from build123d import *

# Parameters (mm, degrees)
SKETCH_1_R          = 22.5
EXTRUDE_1_DEPTH     = 3
SKETCH_2_R          = 22.5
SKETCH_2_R_2        = 21
EXTRUDE_2_DEPTH     = 9
SKETCH_4_R          = 4.1
SKETCH_4_R_2        = 1.5
CUT_EXTRUDE_1_DEPTH = 35.007352146


with BuildPart() as part:
    # 草图1 → 凸台-拉伸1 (new body)
    with BuildSketch(Plane.XY):
        Circle(SKETCH_1_R)
    extrude(amount=EXTRUDE_1_DEPTH)

    # 草图2 → 凸台-拉伸2 (add)
    with BuildSketch(Plane.XY.offset(3)):
        Circle(SKETCH_2_R)
        Circle(SKETCH_2_R_2, mode=Mode.SUBTRACT)
    extrude(amount=EXTRUDE_2_DEPTH)

    # 草图4 → 切除-拉伸1 (cut, through all)
    with BuildSketch(Plane(origin=(0, 0, 0), x_dir=(-1, 0, 0), z_dir=(0, 0, -1))):
        Circle(SKETCH_4_R)
        with Locations((0, 6.5)):
            Circle(SKETCH_4_R_2)
        with Locations((0, -6.5)):
            Circle(SKETCH_4_R_2)
    extrude(amount=-CUT_EXTRUDE_1_DEPTH, mode=Mode.SUBTRACT)


solid = part.part
For this review, take the finished solid that the model builds, in its own axes (mm). A direction names the side the tool comes from. Round coordinates to 2 decimals unless told otherwise and drop trailing zeros. Loops run counter-clockwise (first coordinate to the right, second up) from the corner with the lowest first, then second, coordinate; pieces in that order, holes last. Notation, with made-up numbers: (5, -35) - (20, -35) arc R22 ccw to (20, -8) - close; hole circle Ø7 at (-1.75, 69.25). An arc over 180 degrees is marked (long way). Answer as CSV lines item,"result".
(1) Wall thickness on line 1 (Y direction, x = 0, z = 0.7); line 2 (Z direction, x = 0, y = -12); line 3 (Y direction, x = 0, z = 7.75): over which ranges is each line inside the solid? List them lowest first.
Checked values:
line 1,"y = -22.5 to -8, -5 to -4.1, 4.1 to 5, 8 to 22.5"
line 2,"z = 0 to 3"
line 3,"y = -22.5 to -21, 21 to 22.5"
(2) Consider section A-A on y = 0. Give the boundary of the cut face in (x, z).
Checked values:
outline,"(-22.5, 0) - (-4.1, 0) - (-4.1, 3) - (-21, 3) - (-21, 12) - (-22.5, 12) - close; (4.1, 0) - (22.5, 0) - (22.5, 12) - (21, 12) - (21, 3) - (4.1, 3) - close"
(3) Insertion check: P1, Ø6, axis at x = -3.5, z = 8, coming from the -Y side; P2, Ø6, axis at y = 7.5, z = 6.5, coming from the -X side; P3, Ø1, axis at x = 3, z = 8, coming from the -Y side. Each pin has a flat end and moves straight along its axis. Give the tip position at first contact, or say it passes through.
Checked values:
P1,"stops at y = -22.49"
P2,"stops at x = -22.05"
P3,"stops at y = -22.36"
(4) Tool access review of faces 4 (the face through (4.4, 0.3, 3)), 5 (the face through (0, 5, 1)): name each direction out of +Z, -Z, +X, -X, +Y, -Y from which nothing blocks a thin tool from reaching the whole face with its end or side.
Checked values:
face 4,"+Z"
face 5,"+Z, -Z"
(5) Consider section B-B on x = 0. Give the boundary of the cut face in (y, z), then the cut area to 3 significant figures.
Checked values:
outline,"(-22.5, 0) - (-8, 0) - (-8, 3) - (-21, 3) - (-21, 12) - (-22.5, 12) - close; (-5, 0) - (-4.1, 0) - (-4.1, 3) - (-5, 3) - close; (4.1, 0) - (5, 0) - (5, 3) - (4.1, 3) - close; (8, 0) - (22.5, 0) - (22.5, 12) - (21, 12) - (21, 3) - (8, 3) - close"
area,"119 mm2"
(6) Consider section D-D on y = 14. Give the boundary of the cut face in (x, z).
Checked values:
outline,"(-17.61, 0) - (17.61, 0) - (17.61, 12) - (15.65, 12) - (15.65, 3) - (-15.65, 3) - (-15.65, 12) - (-17.61, 12) - close"
(7) Consider section C-C on z = 1. Give the boundary of the cut face in (x, y).
Checked values:
outline,"circle Ø45 at (0, 0); hole circle Ø8.2 at (0, 0); hole circle Ø3 at (0, -6.5); hole circle Ø3 at (0, 6.5)"
(8) Mouldability with a two-part tool opening along Y and no side actions: class faces 1 (the face through (0, -8, 1)), 2 (the face through (-0.3, -4.7, 0)), 3 (the face through (10.382, -19.961, 5.916)) as +Y half, -Y half, draft (parallel to the pull), parting line (faces both ways), or undercut.
Checked values:
face 1,"undercut"
face 2,"draft"
face 3,"parting line"
